```python
from build123d import *

# Parameters (mm, degrees)
SKETCH_1_W          = 21.5
SKETCH_1_H          = 14.5
EXTRUDE_1_DEPTH     = 10
SKETCH_2_W          = 4.5
SKETCH_2_H          = 4.2
CUT_EXTRUDE_1_DEPTH = 3
SKETCH_2_3_R        = 2.5
SKETCH_2_3_W        = 4.6
SKETCH_2_3_H        = 4.6
CUT_EXTRUDE_2_DEPTH = 2
SKETCH_2_4_R        = 3
SKETCH_2_4_R_2      = 2.5
CUT_EXTRUDE_3_DEPTH = 1
SKETCH_3_W          = 7
SKETCH_3_H          = 7
EXTRUDE_2_DEPTH     = 0.8
SKETCH_4_R          = 0.6
SKETCH_4_W          = 8
SKETCH_4_H          = 3.5
EXTRUDE_3_DEPTH     = 0.6
FILLET_1_R          = 0.4
SKETCH_5_R          = 0.35
CUT_EXTRUDE_4_DEPTH = 0.2
FILLET_2_R          = 0.1


with BuildPart() as part:
    # 草图1 → 凸台-拉伸1 (new body)
    with BuildSketch(Plane(origin=(0, 0, 0), x_dir=(1, 0, 0), z_dir=(0, 1, 0))):
        Rectangle(SKETCH_1_W, SKETCH_1_H)
    extrude(amount=EXTRUDE_1_DEPTH)

    # 草图2 → 切除-拉伸1 (cut)
    with BuildSketch(Plane.XY.offset(7.25)):
        with Locations((-6.9, 5)):
            Rectangle(SKETCH_2_W, SKETCH_2_H)
    extrude(amount=-CUT_EXTRUDE_1_DEPTH, mode=Mode.SUBTRACT)

    # 草图2<3> → 切除-拉伸2 (cut)
    with BuildSketch(Plane.XY.offset(7.25)):
        with Locations((0, 5)):
            Circle(SKETCH_2_3_R)
        with Locations((6.9, 5)):
            Rectangle(SKETCH_2_3_W, SKETCH_2_3_H)
    extrude(amount=-CUT_EXTRUDE_2_DEPTH, mode=Mode.SUBTRACT)

    # 草图2<4> → 切除-拉伸3 (cut)
    with BuildSketch(Plane.XY.offset(7.25)):
        with Locations((0, 5)):
            Circle(SKETCH_2_4_R)
        with Locations((0, 5)):
            Circle(SKETCH_2_4_R_2, mode=Mode.SUBTRACT)
    extrude(amount=-CUT_EXTRUDE_3_DEPTH, mode=Mode.SUBTRACT)

    # 草图3 → 凸台-拉伸2 (add)
    with BuildSketch(Plane(origin=(0, 10, 0), x_dir=(1, 0, 0), z_dir=(0, 1, 0))):
        with Locations((5.98, -2.48)):
            Rectangle(SKETCH_3_W, SKETCH_3_H)
    extrude(amount=EXTRUDE_2_DEPTH)

    # 草图4 → 凸台-拉伸3 (add)
    with BuildSketch(Plane(origin=(0, 10, 0), x_dir=(1, 0, 0), z_dir=(0, 1, 0))):
        with Locations((-9.75, -6.25)):
            Circle(SKETCH_4_R)
        with Locations((9.75, 6.25)):
            Circle(SKETCH_4_R)
        with Locations((-6.55, 5)):
            Rectangle(SKETCH_4_W, SKETCH_4_H)
    extrude(amount=EXTRUDE_3_DEPTH)

    # 圆角1
    fillet_1_edges = [part.edges().sort_by_distance(p)[0] for p in [
        (-10.35, 10.6, 6.25),
        (9.15, 10.6, -6.25),
    ]]
    fillet(fillet_1_edges, radius=FILLET_1_R)

    # 草图5 → 切除-拉伸4 (cut)
    with BuildSketch(Plane.XY.offset(5.25)):
        with Locations((0, 5)):
            Circle(SKETCH_5_R)
    extrude(amount=-CUT_EXTRUDE_4_DEPTH, mode=Mode.SUBTRACT)

    # 圆角2
    fillet_2_edges = [part.edges().sort_by_distance(p)[0] for p in [
        (-4.65, 5, 7.25),
        (-4.65, 7.1, 5.75),
        (-6.9, 2.9, 4.25),
        (-4.65, 2.9, 5.75),
        (-9.15, 5, 4.25),
        (-9.15, 2.9, 5.75),
        (-6.9, 7.1, 7.25),
        (-9.15, 7.1, 5.75),
        (-4.65, 5, 4.25),
        (-6.9, 7.1, 4.25),
        (-9.15, 5, 7.25),
        (-6.9, 2.9, 7.25),
        (6.9, 2.7, 5.25),
        (9.2, 2.7, 6.25),
        (4.6, 5, 5.25),
        (4.6, 2.7, 6.25),
        (6.9, 7.3, 7.25),
        (4.6, 7.3, 6.25),
        (9.2, 5, 7.25),
        (9.2, 7.3, 6.25),
        (6.9, 7.3, 5.25),
        (9.2, 5, 5.25),
        (6.9, 2.7, 7.25),
        (4.6, 5, 7.25),
        (-10.75, 5, -7.25),
        (10.75, 5, -7.25),
        (10.75, 5, 7.25),
        (-10.75, 5, 7.25),
    ]]
    fillet(fillet_2_edges, radius=FILLET_2_R)


solid = part.part
```
Work out the finished part from the listing and answer in its coordinate system (mm). A direction names the side the tool comes from. Round coordinates to 2 decimals unless told otherwise and drop trailing zeros. Loops run counter-clockwise (first coordinate to the right, second up) from the corner with the lowest first, then second, coordinate; pieces in that order, holes last. Notation, with made-up numbers: M 30,33 L 35,33 A8 ccw 35,46 Z; hole C 58.5,86.5 d11. An arc over 180 degrees is marked long. One line per question, with ' | ' between items.
Q1. Each of these flat-tipped pins is pushed along its axis until it touches: pin 1 Ø0.5 at (x, y) = (-6.5, 10.5) entering from +Z; pin 2 Ø1.8 at (x, z) = (-5.5, -6) entering from +Y; pin 3 Ø2 at (x, y) = (8, 5.5) entering from +Z. Where does it stop, or does it pass through?
Conclusion:
pin 1: stops at z = -3.25 | pin 2: stops at y = 10.6 | pin 3: stops at z = 5.25
Q2. Find section D-D, the plane x = 7.25. Give the vertices of the cut face in (y, z).
Conclusion:
outline: M 0,-7.25 L 10,-7.25 L 10,-1.02 L 10.8,-1.02 L 10.8,5.98 L 10,5.98 L 10,7.25 L 7.4,7.25 A0.1 ccw 7.3,7.15 L 7.3,5.35 A0.1 cw 7.2,5.25 L 2.8,5.25 A0.1 cw 2.7,5.35 L 2.7,7.15 A0.1 ccw 2.6,7.25 L 0,7.25 Z
Q3. A tool of negligible diameter and unlimited length cuts with its end or side. For faces 1 (the flat face through (-7, 10.6, -5)), 2 (the flat face through (9.48, 10.4, 2.5)), 3 (the flat face through (7, 7.3, 6)), from which of +Z, -Z, +X, -X, +Y, -Y can it reach the whole face along a straight path? Write none if from no direction.
Conclusion:
face 1: +Z, -Z, +X, -X, +Y | face 2: +Z, +X, +Y | face 3: +Z
Q4. Find section B-B, the plane z = -4.5. Give the vertices of the cut face in (x, y).
Conclusion:
outline: M -10.75,0 L 10.75,0 L 10.75,10 L -2.55,10 L -2.55,10.6 L -10.55,10.6 L -10.55,10 L -10.75,10 Z
Q5. Find section A-A, the plane x = 0. Give the vertices of the cut face in (y, z), then the cut area to 3 significant figures.
Conclusion:
outline: M 0,-7.25 L 10,-7.25 L 10,7.25 L 8,7.25 L 8,6.25 L 7.5,6.25 L 7.5,5.25 L 5.35,5.25 L 5.35,5.05 L 4.65,5.05 L 4.65,5.25 L 2.5,5.25 L 2.5,6.25 L 2,6.25 L 2,7.25 L 0,7.25 Z | area: 134 mm2
Q6. Consider line 1 along Y through (x, z) = (0, 6.95); line 2 along Z through (x, y) = (-0.75, 2.25); line 3 along Y through (x, z) = (-3.75, -3). Determine where each line is inside the solid, lowest interval first. Write a range as from..to.
Conclusion:
line 1: y = 0..2, 8..10 | line 2: z = -7.25..6.25 | line 3: y = 0..10
Q7. The mould has two halves that part along Y. Classify faces 4 (the flat face through (10.75, 5, 0)), 5 (the flat face through (-7, 7.1, 6)), 6 (the flat face through (0, 0, 0)): +Y half, -Y half, draft (parallel to the pull), parting line (faces both ways), or undercut.
Conclusion:
face 4: draft | face 5: undercut | face 6: -Y half
